from build123d import *

# Parameters (mm, degrees)
SKETCH1_R      = 5
EXTRUDE1_DEPTH = 61.6
SKETCH2_R      = 3
EXTRUDE2_DEPTH = 5.2
EXTRUDE3_START = 14.2
SKETCH3_R      = 3
EXTRUDE3_DEPTH = 14.2
SKETCH5_R      = 1.5
EXTRUDE5_DEPTH = 2


with BuildPart() as part:
    # Sketch1 → Extrude1 (new body)
    with BuildSketch(Plane.XY):
        with Locations(Location((0, 0, 0), (0, 0, 180))):
            Circle(SKETCH1_R)
    extrude(amount=EXTRUDE1_DEPTH)

    # Sketch2 → Extrude2 (add)
    with BuildSketch(Plane.XY.offset(61.6)):
        Circle(SKETCH2_R)
    extrude(amount=EXTRUDE2_DEPTH)

    # Sketch3 → Extrude3 (add)
    with BuildSketch(Plane(origin=(0, 0, 0), x_dir=(-1, 0, 0), z_dir=(0, 0, -1)).offset(EXTRUDE3_START)):
        with Locations(Location((0, 0, 0), (0, 0, 180))):
            Circle(SKETCH3_R)
    extrude(amount=-EXTRUDE3_DEPTH)

    # Sketch5 → Extrude5 (cut)
    with BuildSketch(Plane(origin=(0, 3, 0), x_dir=(-1, 0, 0), z_dir=(0, 1, 0))):
        with Locations(Location((0, -4.55, 0), (0, 0, 90))):
            Circle(SKETCH5_R)
    extrude(amount=-EXTRUDE5_DEPTH, mode=Mode.SUBTRACT)


solid = part.part
Geometry: final body of the model. Coordinates: model frame, mm. A direction names the side the tool comes from. Coordinates: 2 decimals unless noted, no trailing zeros. Loops run counter-clockwise (first coordinate to the right, second up) from the corner with the lowest first, then second, coordinate; pieces in that order, holes last. Notation, with made-up numbers: M -22,34 L -7,34 A8 cw -7,44 Z; hole C -7,-13.5 d4. An arc over 180 degrees is marked long. One line per item, written item: value. Start each with the question number.
1) Cut plane D-D (y = -4.25). Return loops of the section in (x, z).
2) Cut plane C-C (z = 14). Return loops of the section in (x, y).
3) Material intervals for L1, parallel to Z at x = 0, y = 2.25; L2, parallel to Z at x = 3, y = -0.75; L3, parallel to X at y = 2.3, z = -4.55, sorted ascending. Write a range as from..to.
4) Pin query (flat end, axial travel): P1, Ø3.5, axis at x = 0, z = -4.5, coming from the +Y side; P2, Ø5, axis at x = 3, z = 50.5, coming from the +Y side; P3, Ø6, axis at y = -4, z = 27, coming from the +X side. Return the tip coordinate at first contact, or that it passes through.
5) Cut plane A-A (x = 0). Return loops of the section in (y, z), then the cut area to 3 significant figures.
6) Draft query along Z for faces 1 (the flat face through (0, 0, 66.8)), 2 (the cylindrical face through (5, 0, 30)), 3 (the flat face through (0, 1, -5)). Return one class per face: released by +Z, released by -Z, zero draft, split by the parting line, or undercut.
7) Reachability of faces 4 (the cylindrical face through (-0.575, 2.014, -3.164)), 5 (the cylindrical face through (0, -3, -7)), 6 (the flat face through (0.1, 3.3, 61.6)) from +Z, -Z, +X, -X, +Y, -Y: full face, straight path, thin tool, end or side. Return the list, or none.
8) Cut plane B-B (y = 0). Return loops of the section in (x, z).
Evaluation:
1. outline: M -2.63,0 L 2.63,0 L 2.63,61.6 L -2.63,61.6 Z
2. outline: C 0,0 d10
3. L1: -14.2..-6.05, -3.05..66.8
3. L2: 0..61.6
3. L3: -1.93..-1.5, 1.5..1.93
4. P1: y = 3
4. P2: y = 4.97
4. P3: x = 4.9
5. outline: M -5,0 L -3,0 L -3,-14.2 L 3,-14.2 L 3,-6.05 L 1,-6.05 L 1,-3.05 L 3,-3.05 L 3,0 L 5,0 L 5,61.6 L 3,61.6 L 3,66.8 L -3,66.8 L -3,61.6 L -5,61.6 Z
5. area: 726 mm^2
6. face 1: released by +Z
6. face 2: zero draft
6. face 3: undercut
7. face 4: +Y
7. face 5: -Z
7. face 6: +Z
8. outline: M -5,0 L -3,0 L -3,-14.2 L 3,-14.2 L 3,0 L 5,0 L 5,61.6 L 3,61.6 L 3,66.8 L -3,66.8 L -3,61.6 L -5,61.6 Z
